from build123d import *

# Parameters (mm, degrees)
SKETCH_1_W          = 47.5
SKETCH_1_H          = 27
EXTRUDE_1_DEPTH     = 4
SKETCH_5_R          = 13.25
EXTRUDE_2_DEPTH     = 4
SKETCH_6_R          = 6
EXTRUDE_3_DEPTH     = 3.5
SKETCH_7_R          = 4
CUT_EXTRUDE_1_DEPTH = 56.834577101
SKETCH_8_R          = 2.5
CUT_EXTRUDE_2_DEPTH = 56.149796011
CUT_EXTRUDE_3_DEPTH = 56.149796011
FILLET_1_R          = 3


with BuildPart() as part:
    # 草图1 → 凸台-拉伸1 (new body)
    with BuildSketch(Plane(origin=(0, 0, 0), x_dir=(0, 0, -1), z_dir=(1, 0, 0))):
        with Locations((23.75, 13.5)):
            Rectangle(SKETCH_1_W, SKETCH_1_H)
    extrude(amount=EXTRUDE_1_DEPTH)

    # 草图5 → 凸台-拉伸2 (add)
    with BuildSketch(Plane.ZY):
        with Locations((-23.75, 13.5)):
            Circle(SKETCH_5_R)
    extrude(amount=EXTRUDE_2_DEPTH)

    # 草图6 → 凸台-拉伸3 (add)
    with BuildSketch(Plane.ZY.offset(4)):
        with Locations((-23.75, 13.5)):
            Circle(SKETCH_6_R)
    extrude(amount=EXTRUDE_3_DEPTH)

    # 草图7 → 切除-拉伸1 (cut, through all)
    with BuildSketch(Plane.ZY.offset(7.5)):
        with Locations((-23.75, 13.5)):
            Circle(SKETCH_7_R)
    extrude(amount=-CUT_EXTRUDE_1_DEPTH, mode=Mode.SUBTRACT)

    # 草图8 → 切除-拉伸2 (cut, through all)
    with BuildSketch(Plane.ZY):
        with Locations((-42.25, 13.5)):
            Circle(SKETCH_8_R)
        with Locations((-5.25, 13.5)):
            Circle(SKETCH_8_R)
    extrude(amount=-CUT_EXTRUDE_2_DEPTH, mode=Mode.SUBTRACT)

    # 草图9 → 切除-拉伸3 (cut, through all)
    with BuildSketch(Plane.ZY):
        Polygon((-47.5, 9), (-30.5, 0), (-47.5, 0), align=None)
        Polygon((-47.5, 18), (-30.5, 27), (-47.5, 27), align=None)
        Polygon((0, 0), (-17, 0), (0, 9), align=None)
        Polygon((0, 18), (0, 27), (-17, 27), align=None)
    extrude(amount=-CUT_EXTRUDE_3_DEPTH, mode=Mode.SUBTRACT)

    # 圆角1
    fillet_1_edges = [part.edges().sort_by_distance(p)[0] for p in [
        (2, 9, -47.5),
        (2, 0, -30.5),
        (2, 18, -47.5),
        (2, 27, -30.5),
        (2, 9, 0),
        (2, 0, -17),
        (2, 18, 0),
        (2, 27, -17),
    ]]
    fillet(fillet_1_edges, radius=FILLET_1_R)


solid = part.part
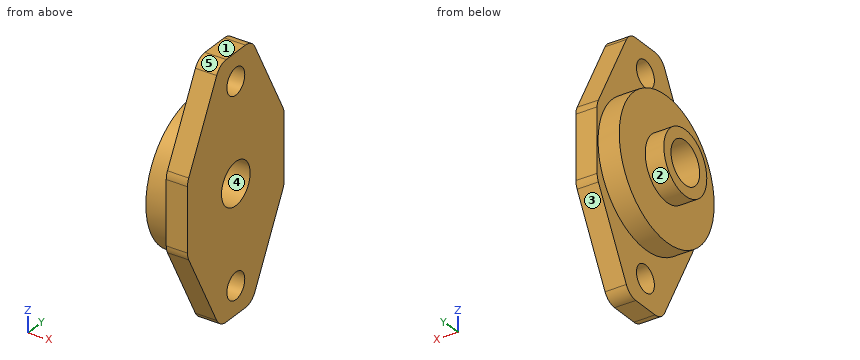
Geometry check sheet. Reference: the model listing, model coordinates, mm. Face numbers are marked on the shaded views. A direction names the side the tool comes from. Give positions to 0.01 mm unless a question says otherwise; leave off trailing zeros. Order: outer loops, then holes, each group sorted by start corner. A loop starts at its lowest first (then second) coordinate and runs counter-clockwise, first axis right, second up. Notation, with made-up numbers: M -38.5,85 L 6.5,85 A33 cw 6.5,121 Z; hole C 88.5,4 d6. An arc over 180 degrees is marked long. Use a Markdown table: item, result.
Item 1: Section check B-B (x = 2.75). Record the cut outline in (y, z), and give its area (3 significant figures).
Answers follow:
| item | result |
|---|---|
| outline | M 0,-29.75 A3 ccw 0.35,-31.16 L 8.15,-45.9 A3 ccw 10.81,-47.5 L 16.19,-47.5 A3 ccw 18.85,-45.9 L 26.65,-31.16 A3 ccw 27,-29.75 L 27,-17.75 A3 ccw 26.65,-16.34 L 18.85,-1.6 A3 ccw 16.19,0 L 10.81,0 A3 ccw 8.15,-1.6 L 0.35,-16.34 A3 ccw 0,-17.75 Z; hole C 13.5,-23.75 d8; hole C 13.5,-42.25 d5; hole C 13.5,-5.25 d5 |
| area | 885 mm2 |
Item 2: Section check A-A (y = 13.5). Record the cut outline in (x, z), and give its area (3 significant figures).
Answers follow:
| item | result |
|---|---|
| outline | M -7.5,-29.75 L -4,-29.75 L -4,-37 L 0,-37 L 0,-39.75 L 4,-39.75 L 4,-27.75 L -7.5,-27.75 Z; M -7.5,-19.75 L 4,-19.75 L 4,-7.75 L 0,-7.75 L 0,-10.5 L -4,-10.5 L -4,-17.75 L -7.5,-17.75 Z; M 0,-47.5 L 4,-47.5 L 4,-44.75 L 0,-44.75 Z; M 0,-2.75 L 4,-2.75 L 4,0 L 0,0 Z |
| area | 206 mm2 |
Item 3: Section check C-C (z = -26). Record the cut outline in (x, y), and give its area (3 significant figures).
Answers follow:
| item | result |
|---|---|
| outline | M -7.5,7.94 L -4,7.94 L -4,0.44 L 0,0.44 L 0,0 L 4,0 L 4,10.19 L -7.5,10.19 Z; M -7.5,16.81 L 4,16.81 L 4,27 L 0,27 L 0,26.56 L -4,26.56 L -4,19.06 L -7.5,19.06 Z |
| area | 175 mm2 |
Item 4: Tool access check on the marked faces 1 and 2. Record the directions out of +Z, -Z, +X, -X, +Y, -Y that give a thin tool (end or side, any length) a straight path to the whole face; none if there is none.
Answers follow:
| item | result |
|---|---|
| face 1 | +Z, +X, -X, +Y, -Y |
| face 2 | -X |
Item 5: Draft check along Y on the marked faces 3, 4 and 5. Enter one of: +Y half, -Y half, draft (parallel to the pull), parting line (faces both ways), or undercut.
Answers follow:
| item | result |
|---|---|
| face 3 | +Y half |
| face 4 | undercut |
| face 5 | -Y half |
Item 6: Depth check by flat-ended pin: P1, Ø6, axis at x = 2.5, z = -42, coming from the +Y side; P2, Ø3, axis at x = 1.5, z = -6.5, coming from the -Y side; P3, Ø8, axis at y = 13.5, z = -42.25, coming from the -X side; P4, Ø4, axis at y = 13.5, z = -5.25, coming from the +X side. Enter the tip coordinate at first touch or a pass-through.
Answers follow:
| item | result |
|---|---|
| P1 | stops at y = 22.5 |
| P2 | stops at y = 4.76 |
| P3 | stops at x = 0 |
| P4 | passes through |
Item 7: Material ranges on line 1 along Y through (x, z) = (-2.25, -23.75); line 2 along X through (y, z) = (15.25, -9.5); line 3 along X through (y, z) = (9.75, -15), recorded low to high.
Answers follow:
| item | result |
|---|---|
| line 1 | y = 0.25 to 9.5, 17.5 to 26.75 |
| line 2 | x = 0 to 4 |
| line 3 | x = -4 to 4 |
Item 8: Section check D-D (y = 22.75). Record the cut outline in (x, z).
Answers follow:
| item | result |
|---|---|
| outline | M -4,-33.24 L 0,-33.24 L 0,-38.53 L 4,-38.53 L 4,-8.97 L 0,-8.97 L 0,-14.26 L -4,-14.26 Z |
